```python
from build123d import *

# Parameters (mm, degrees)
EXTRUDE_1_DEPTH     = 12
HOLE_WIZARD_M5_1_D  = 4.2
SKETCH_5_R          = 10
CUT_EXTRUDE_1_DEPTH = 114.771701227
CHAMFER_1_SIZE      = 0.5


with BuildPart() as part:
    # 스케치1 → 보스-돌출1 (new body)
    with BuildSketch(Plane(origin=(0, 0, 0), x_dir=(1, 0, 0), z_dir=(0, 1, 0))):
        Polygon((0, 75), (5, 80), (75, 80), (80, 75), (80, 5), (75, 0), (5, 0), (0, 5), align=None)
    extrude(amount=EXTRUDE_1_DEPTH)

    # M5 나사 구멍1 (through all)
    with Locations(Plane(origin=(0, 12, 0), x_dir=(1, 0, 0), z_dir=(0, 1, 0))):
        with Locations((6.765981284, 73.234018716), (40, 62.5), (73.234018716, 73.234018716), (62.5, 40), (40, 17.5), (17.5, 40), (6.765981284, 6.765981284), (73.234018716, 6.765981284)):
            Hole(HOLE_WIZARD_M5_1_D / 2)

    # 스케치5 → 컷-돌출1 (cut, through all)
    with BuildSketch(Plane(origin=(0, 12, 0), x_dir=(1, 0, 0), z_dir=(0, 1, 0))):
        with Locations(Location((40, 40, 0), (0, 0, 270))):
            Circle(SKETCH_5_R)
    extrude(amount=-CUT_EXTRUDE_1_DEPTH, mode=Mode.SUBTRACT)

    # 모따기1
    chamfer_1_edges = [part.edges().sort_by_distance(p)[0] for p in [
        (40, 0, -50),
        (40, 12, -50),
    ]]
    chamfer(chamfer_1_edges, length=CHAMFER_1_SIZE)


solid = part.part
```
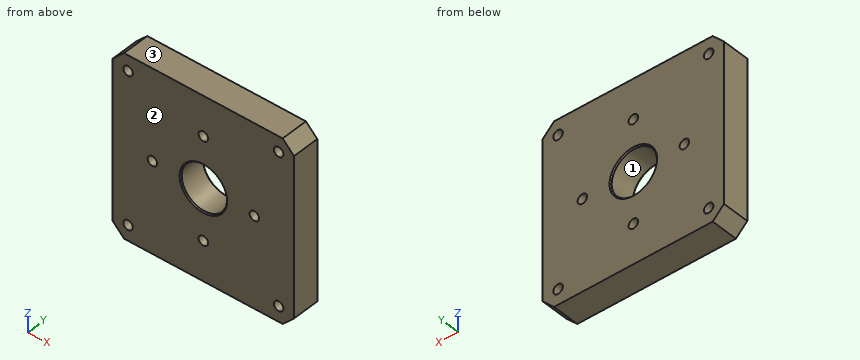
CAD build for the part. Positions are in the model's coordinates, mm. Face numbers are marked on the shaded views. Coordinates: 2 decimals unless noted, no trailing zeros. Write each loop counter-clockwise with the first axis right and the second up, starting at its lowest first coordinate (ties: lowest second). Pieces come first, ordered by that corner, then holes. Notation, with made-up numbers: (5, 73) -> (55, 73) arc R30 ccw to (55, 103) -> close; hole circle Ø2 at (-25, 55.5). An arc over 180 degrees is marked (long way). Return JSON: item names as keys, results as strings. Group by question number.
Q1. Cut at C-C, the plane z = -40. Give the cut face in (x, y), then the cut area to 3 significant figures.
Q2. Drill centre lines: line 1 (X direction, y = 5.25, z = -40); line 2 (X direction, y = 8.25, z = -62.5); line 3 (Z direction, x = 40.5, y = 3). Where is each one in solid material? Low to high.
Q3. Cut at B-B, the plane x = 17.5. Give the cut face in (y, z).
Q4. Cut at A-A, the plane z = -17.5. Give the cut face in (x, y), then the cut area to 3 significant figures.
Q5. Pull direction Z, two halves, no side cores. Call the marked faces 1, 2 and 3: released by +Z, released by -Z, zero draft, split by the parting line, or undercut.
Q6. Cut at D-D, the plane x = 40. Give the cut face in (y, z), then the cut area to 3 significant figures.
Q7. Flat gauge pins, fed straight in: pin 1 (6.5 mm diameter, centred on x = 62.5, z = -40, fed in from +Y); pin 2 (3.5 mm diameter, centred on x = 73.23, z = -73.23, fed in from +Y). Where does each tip first touch, or does it go through?
Returned:
{
 "1": {"outline": "(0, 0) -> (15.4, 0) -> (15.4, 12) -> (0, 12) -> close; (19.6, 0) -> (29.5, 0) -> (30, 0.5) -> (30, 11.5) -> (29.5, 12) -> (19.6, 12) -> close; (50, 0.5) -> (50.5, 0) -> (60.4, 0) -> (60.4, 12) -> (50.5, 12) -> (50, 11.5) -> close; (64.6, 0) -> (80, 0) -> (80, 12) -> (64.6, 12) -> close", "area": "619 mm2"},
 "2": {"line 1": "x = 0 to 15.4, 19.6 to 30, 50 to 60.4, 64.6 to 80", "line 2": "x = 0 to 37.9, 42.1 to 80", "line 3": "z = -80 to -64.54, -60.46 to -49.99, -30.01 to -19.54, -15.46 to 0"},
 "3": {"outline": "(0, -80) -> (12, -80) -> (12, -42.1) -> (0, -42.1) -> close; (0, -37.9) -> (12, -37.9) -> (12, 0) -> (0, 0) -> close"},
 "4": {"outline": "(0, 0) -> (37.9, 0) -> (37.9, 12) -> (0, 12) -> close; (42.1, 0) -> (80, 0) -> (80, 12) -> (42.1, 12) -> close", "area": "910 mm2"},
 "5": {"face 1": "undercut", "face 2": "zero draft", "face 3": "released by +Z"},
 "6": {"outline": "(0, -80) -> (12, -80) -> (12, -64.6) -> (0, -64.6) -> close; (0, -60.4) -> (12, -60.4) -> (12, -50.5) -> (11.5, -50) -> (0.5, -50) -> (0, -50.5) -> close; (0, -29.5) -> (0.5, -30) -> (11.5, -30) -> (12, -29.5) -> (12, -19.6) -> (0, -19.6) -> close; (0, -15.4) -> (12, -15.4) -> (12, 0) -> (0, 0) -> close", "area": "619 mm2"},
 "7": {"pin 1": "stops at y = 12", "pin 2": "passes through"}
}
